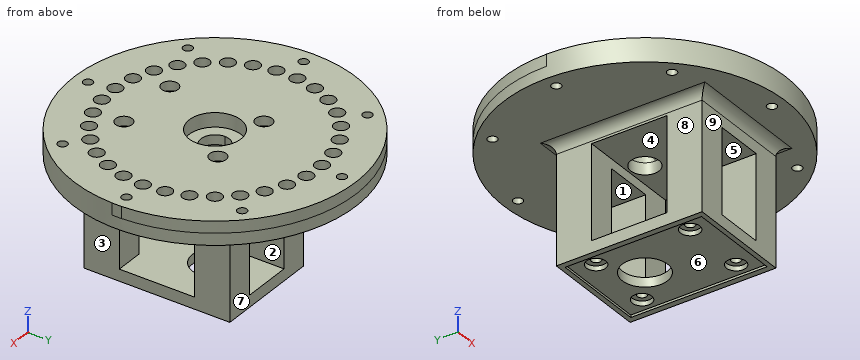
from build123d import *

# Parameters (mm, degrees)
SKETCH1_R               = 3
SKETCH1_R_2             = 11
BOSS_EXTRUDE1_DEPTH     = 5
BOSS_EXTRUDE2_START     = 5
SKETCH2_R               = 60
SKETCH2_R_2             = 6
BOSS_EXTRUDE2_DEPTH     = 5
SKETCH3_R               = 2
CUT_EXTRUDE1_DEPTH      = 35
CUT_EXTRUDE2_START      = -1
SKETCH4_R               = 11
CUT_EXTRUDE2_DEPTH      = 1
CUT_EXTRUDE3_DEPTH      = 87.852680842
CUT_EXTRUDE3_DEPTH_BACK = 87.852680842
SKETCH5_R               = 2
SKETCH6_W               = 45
SKETCH6_H               = 62
BOSS_EXTRUDE3_DEPTH     = 50
CUT_EXTRUDE4_START      = -40
SKETCH7_R               = 2
SKETCH7_R_2             = 6
CUT_EXTRUDE4_DEPTH      = 40
CUT_EXTRUDE5_DEPTH      = 88
CUT_EXTRUDE5_DEPTH_BACK = 5
SKETCH8_R               = 9.6
SKETCH9_W               = 40
SKETCH9_H               = 32
CUT_EXTRUDE6_DEPTH      = 71
SKETCH10_R              = 3.5
CUT_EXTRUDE7_DEPTH      = 4
FILLET1_R               = 4
SKETCH11_W              = 40
SKETCH11_H              = 58
CUT_EXTRUDE8_DEPTH      = 1
SKETCH12_W              = 21
SKETCH12_H              = 36
CUT_EXTRUDE9_DEPTH      = 88
CUT_EXTRUDE10_START     = -88
SKETCH13_R              = 2
CUT_EXTRUDE10_DEPTH     = 88
CUT_EXTRUDE11_START     = -10
SKETCH14_R              = 82.644594736
SKETCH14_R_2            = 60
CUT_EXTRUDE11_DEPTH     = 10
SKETCH15_R              = 4.1
CUT_EXTRUDE12_DEPTH     = 2


with BuildPart() as part:
    # Sketch1 → Boss-Extrude1 (new body)
    with BuildSketch(Plane.XY):
        with BuildLine():
            ThreePointArc((59.966830941, 1.994789941), (-60, 0), (59.966830941, -1.994789941))
            ThreePointArc((59.966830941, -1.994789941), (61.995065687, 0), (59.966830941, 1.994789941))
        make_face()
        with Locations((44, 0)):
            Circle(SKETCH1_R, mode=Mode.SUBTRACT)
        with Locations((43.099317415, -8.857134884)):
            Circle(SKETCH1_R, mode=Mode.SUBTRACT)
        with Locations((40.434143711, -17.351657625)):
            Circle(SKETCH1_R, mode=Mode.SUBTRACT)
        with Locations((36.113591413, -25.135801464)):
            Circle(SKETCH1_R, mode=Mode.SUBTRACT)
        with Locations((30.314544439, -31.890882638)):
            Circle(SKETCH1_R, mode=Mode.SUBTRACT)
        with Locations((23.274416454, -37.34034733)):
            Circle(SKETCH1_R, mode=Mode.SUBTRACT)
        with Locations((15.281431125, -41.261093814)):
            Circle(SKETCH1_R, mode=Mode.SUBTRACT)
        with Locations((6.66282221, -43.49260627)):
            Circle(SKETCH1_R, mode=Mode.SUBTRACT)
        with Locations((-2.228563429, -43.943526316)):
            Circle(SKETCH1_R, mode=Mode.SUBTRACT)
        with Locations((-11.028711419, -42.59539323)):
            Circle(SKETCH1_R, mode=Mode.SUBTRACT)
        with Locations((-19.377342669, -39.503399741)):
            Circle(SKETCH1_R, mode=Mode.SUBTRACT)
        with Locations((-26.932663232, -34.794132425)):
            Circle(SKETCH1_R, mode=Mode.SUBTRACT)
        with Locations((-33.385357398, -28.66038924)):
            Circle(SKETCH1_R, mode=Mode.SUBTRACT)
        with Locations((-38.47125111, -21.353286351)):
            Circle(SKETCH1_R, mode=Mode.SUBTRACT)
        with Locations((-41.982127282, -13.171977411)):
            Circle(SKETCH1_R, mode=Mode.SUBTRACT)
        with Locations((-43.774250229, -4.451406167)):
            Circle(SKETCH1_R, mode=Mode.SUBTRACT)
        with Locations((-43.774250229, 4.451406167)):
            Circle(SKETCH1_R, mode=Mode.SUBTRACT)
        with Locations((-41.982127282, 13.171977411)):
            Circle(SKETCH1_R, mode=Mode.SUBTRACT)
        with Locations((-38.47125111, 21.353286351)):
            Circle(SKETCH1_R, mode=Mode.SUBTRACT)
        with Locations((-33.385357398, 28.66038924)):
            Circle(SKETCH1_R, mode=Mode.SUBTRACT)
        with Locations((-26.932663232, 34.794132425)):
            Circle(SKETCH1_R, mode=Mode.SUBTRACT)
        with Locations((-19.377342669, 39.503399741)):
            Circle(SKETCH1_R, mode=Mode.SUBTRACT)
        with Locations((-11.028711419, 42.59539323)):
            Circle(SKETCH1_R, mode=Mode.SUBTRACT)
        with Locations((-2.228563429, 43.943526316)):
            Circle(SKETCH1_R, mode=Mode.SUBTRACT)
        with Locations((6.66282221, 43.49260627)):
            Circle(SKETCH1_R, mode=Mode.SUBTRACT)
        with Locations((15.281431125, 41.261093814)):
            Circle(SKETCH1_R, mode=Mode.SUBTRACT)
        with Locations((23.274416454, 37.34034733)):
            Circle(SKETCH1_R, mode=Mode.SUBTRACT)
        with Locations((30.314544439, 31.890882638)):
            Circle(SKETCH1_R, mode=Mode.SUBTRACT)
        with Locations((36.113591413, 25.135801464)):
            Circle(SKETCH1_R, mode=Mode.SUBTRACT)
        with Locations((40.434143711, 17.351657625)):
            Circle(SKETCH1_R, mode=Mode.SUBTRACT)
        with Locations((43.099317415, 8.857134884)):
            Circle(SKETCH1_R, mode=Mode.SUBTRACT)
        Circle(SKETCH1_R_2, mode=Mode.SUBTRACT)
    extrude(amount=BOSS_EXTRUDE1_DEPTH)

    # Sketch2 → Boss-Extrude2 (add)
    with BuildSketch(Plane(origin=(0, 0, 0), x_dir=(-1, 0, 0), z_dir=(0, 0, -1)).offset(BOSS_EXTRUDE2_START)):
        Circle(SKETCH2_R)
        Circle(SKETCH2_R_2, mode=Mode.SUBTRACT)
    extrude(amount=-BOSS_EXTRUDE2_DEPTH)

    # Sketch3 → Cut-Extrude1 (cut)
    with BuildSketch(Plane.XY.offset(5)):
        with Locations((0, 54)):
            Circle(SKETCH3_R)
        with Locations((38.183766184, 38.183766184)):
            Circle(SKETCH3_R)
        with Locations((54, 0)):
            Circle(SKETCH3_R)
        with Locations((38.183766184, -38.183766184)):
            Circle(SKETCH3_R)
        with Locations((0, -54)):
            Circle(SKETCH3_R)
        with Locations((-38.183766184, -38.183766184)):
            Circle(SKETCH3_R)
        with Locations((-54, 0)):
            Circle(SKETCH3_R)
        with Locations((-38.183766184, 38.183766184)):
            Circle(SKETCH3_R)
    extrude(amount=-CUT_EXTRUDE1_DEPTH, mode=Mode.SUBTRACT)

    # Sketch4 → Cut-Extrude2 (cut)
    with BuildSketch(Plane.XY.offset(CUT_EXTRUDE2_START)):
        Circle(SKETCH4_R)
    extrude(amount=CUT_EXTRUDE2_DEPTH, mode=Mode.SUBTRACT)

    # Sketch5 → Cut-Extrude3 (cut, two sides: drawn at the far end of the back side and taken through both)
    with BuildSketch(Plane(origin=(0, 0, -5), x_dir=(-1, 0, 0), z_dir=(0, 0, -1)).offset(-CUT_EXTRUDE3_DEPTH_BACK)):
        with Locations((-14, 11)):
            Circle(SKETCH5_R)
        with Locations((14, 11)):
            Circle(SKETCH5_R)
        with Locations((14, -29)):
            Circle(SKETCH5_R)
        with Locations((-14, -29)):
            Circle(SKETCH5_R)
    extrude(amount=CUT_EXTRUDE3_DEPTH + CUT_EXTRUDE3_DEPTH_BACK, mode=Mode.SUBTRACT)

    # Sketch6 → Boss-Extrude3 (add)
    with BuildSketch(Plane(origin=(0, 0, -5), x_dir=(-1, 0, 0), z_dir=(0, 0, -1))):
        with Locations((0, -9)):
            Rectangle(SKETCH6_W, SKETCH6_H)
    extrude(amount=BOSS_EXTRUDE3_DEPTH)

    # Sketch7 → Cut-Extrude4 (cut)
    with BuildSketch(Plane.XY.offset(5).offset(CUT_EXTRUDE4_START)):
        with Locations((-14, 11)):
            Circle(SKETCH7_R)
        with Locations(Location((14, 11, 0), (0, 0, 180))):
            Circle(SKETCH7_R)
        with Locations((14, -29)):
            Circle(SKETCH7_R)
        with Locations(Location((-14, -29, 0), (0, 0, 180))):
            Circle(SKETCH7_R)
        Circle(SKETCH7_R_2)
    extrude(amount=CUT_EXTRUDE4_DEPTH, mode=Mode.SUBTRACT)

    # Sketch8 → Cut-Extrude5 (cut, two sides: drawn at the far end of the back side and taken through both)
    with BuildSketch(Plane(origin=(0, 0, -55), x_dir=(-1, 0, 0), z_dir=(0, 0, -1)).offset(-CUT_EXTRUDE5_DEPTH_BACK)):
        Circle(SKETCH8_R)
    extrude(amount=CUT_EXTRUDE5_DEPTH + CUT_EXTRUDE5_DEPTH_BACK, mode=Mode.SUBTRACT)

    # Sketch9 → Cut-Extrude6 (cut)
    with BuildSketch(Plane.ZY.offset(22.5)):
        with Locations((-30, -9)):
            Rectangle(SKETCH9_W, SKETCH9_H)
    extrude(amount=-CUT_EXTRUDE6_DEPTH, mode=Mode.SUBTRACT)

    # Sketch10 → Cut-Extrude7 (cut)
    with BuildSketch(Plane.XY.offset(5)):
        with Locations((-14, 11)):
            Circle(SKETCH10_R)
        with Locations((14, 11)):
            Circle(SKETCH10_R)
        with Locations((-14, -29)):
            Circle(SKETCH10_R)
        with Locations((14, -29)):
            Circle(SKETCH10_R)
    extrude(amount=-CUT_EXTRUDE7_DEPTH, mode=Mode.SUBTRACT)

    # Fillet1
    fillet1_edges = [part.edges().sort_by_distance(p)[0] for p in [
        (-22.5, -9, -5),
        (0, 22, -5),
        (22.5, -9, -5),
        (0, -40, -5),
    ]]
    fillet(fillet1_edges, radius=FILLET1_R)

    # Sketch11 → Cut-Extrude8 (cut)
    with BuildSketch(Plane(origin=(0, 0, -55), x_dir=(-1, 0, 0), z_dir=(0, 0, -1))):
        with Locations((0, -9)):
            Rectangle(SKETCH11_W, SKETCH11_H)
    extrude(amount=-CUT_EXTRUDE8_DEPTH, mode=Mode.SUBTRACT)

    # Sketch12 → Cut-Extrude9 (cut)
    with BuildSketch(Plane.XZ.offset(40)):
        with Locations((0, -32)):
            Rectangle(SKETCH12_W, SKETCH12_H)
    extrude(amount=-CUT_EXTRUDE9_DEPTH, mode=Mode.SUBTRACT)

    # Sketch13 → Cut-Extrude10 (cut)
    with BuildSketch(Plane.XY.offset(1).offset(CUT_EXTRUDE10_START)):
        with Locations(Location((-14, 11, 0), (0, 0, 180))):
            Circle(SKETCH13_R)
        with Locations(Location((14, 11, 0), (0, 0, 180))):
            Circle(SKETCH13_R)
        with Locations(Location((14, -29, 0), (0, 0, 180))):
            Circle(SKETCH13_R)
        with Locations(Location((-14, -29, 0), (0, 0, 180))):
            Circle(SKETCH13_R)
    extrude(amount=CUT_EXTRUDE10_DEPTH, mode=Mode.SUBTRACT)

    # Sketch14 → Cut-Extrude11 (cut)
    with BuildSketch(Plane.XY.offset(5).offset(CUT_EXTRUDE11_START)):
        Circle(SKETCH14_R)
        with Locations(Location((0, 0, 0), (0, 0, 180))):
            Circle(SKETCH14_R_2, mode=Mode.SUBTRACT)
    extrude(amount=CUT_EXTRUDE11_DEPTH, mode=Mode.SUBTRACT)

    # Sketch15 → Cut-Extrude12 (cut)
    with BuildSketch(Plane(origin=(0, 0, -54), x_dir=(-1, 0, 0), z_dir=(0, 0, -1))):
        with Locations((14, 11)):
            Circle(SKETCH15_R)
        with Locations((-14, 11)):
            Circle(SKETCH15_R)
        with Locations((-14, -29)):
            Circle(SKETCH15_R)
        with Locations((14, -29)):
            Circle(SKETCH15_R)
    extrude(amount=-CUT_EXTRUDE12_DEPTH, mode=Mode.SUBTRACT)


solid = part.part
Work out the finished part from the listing and answer in its coordinate system (mm). Face numbers are marked on the shaded views. A direction names the side the tool comes from. Give positions to 0.01 mm unless a question says otherwise; leave off trailing zeros. Order: outer loops, then holes, each group sorted by start corner. A loop starts at its lowest first (then second) coordinate and runs counter-clockwise, first axis right, second up. Notation, with made-up numbers: (81.25, 15) -> (133.25, 15) arc R26 cw to (133.25, 50) -> close; hole circle Ø4 at (86.5, -14.75). An arc over 180 degrees is marked (long way). One line per item, written item: value.
Item 1: Find section A-A, the plane z = -37. Give the vertices of the cut face in (x, y), plus the area to 3 significant figures.
Answer sheet:
outline: (-22.5, -40) -> (-10.5, -40) -> (-10.5, -25) -> (-22.5, -25) -> close; (-22.5, 7) -> (-10.5, 7) -> (-10.5, 22) -> (-22.5, 22) -> close; (10.5, -40) -> (22.5, -40) -> (22.5, -25) -> (10.5, -25) -> close; (10.5, 7) -> (22.5, 7) -> (22.5, 22) -> (10.5, 22) -> close; hole circle Ø4 at (-14, -29); hole circle Ø4 at (-14, 11); hole circle Ø4 at (14, -29); hole circle Ø4 at (14, 11)
area: 670 mm²
Item 2: Find section D-D, the plane z = -7. Give the vertices of the cut face in (x, y), plus the area to 3 significant figures.
Answer sheet:
outline: (-23.04, -40.54) -> (23.04, -40.54) -> (23.04, 22.54) -> (-23.04, 22.54) -> close; hole circle Ø4 at (-14, -29); hole circle Ø4 at (-14, 11); hole circle Ø12 at (0, 0); hole circle Ø4 at (14, -29); hole circle Ø4 at (14, 11)
area: 2,740 mm²
Item 3: Straight lines are drawn through the part: probe 1 along Y at (x, z) = (-14, -26); probe 2 along Y at (x, z) = (-20.5, -37); probe 3 along Z at (x, y) = (-6, -24). For each, find the intervals that lie inside material, in ascending order.
Answer sheet:
probe 1: -40 to -31, -27 to -25, 7 to 9, 13 to 22
probe 2: -40 to -25, 7 to 22
probe 3: -54 to -50, -10 to 5
Item 4: Find section B-B, the plane x = 54. Give the vertices of the cut face in (y, z), plus the area to 3 significant figures.
Answer sheet:
outline: (-26.15, -5) -> (-2, -5) -> (-2, 5) -> (-26.15, 5) -> close; (2, -5) -> (26.15, -5) -> (26.15, 5) -> (2, 5) -> close
area: 483 mm²
Item 5: Flat-ended cylindrical pins translate along their axes: P1, Ø4.5, axis at x = 54, y = 0, coming from the +Z side; P2, Ø3, axis at x = -26, y = -35, coming from the +Z side; P3, Ø4, axis at y = -38, z = -42, coming from the -X side; P4, Ø20, axis at x = -11, z = -22.5, coming from the -Y side. Find the tip coordinate at first contact, or state that the pin passes through.
Answer sheet:
P1: z = 5
P2: z = 0
P3: x = -22.5
P4: y = -40
Item 6: Determine the mould class of the marked faces 1, 2, 3 and 4 for opening direction X: released by +X, released by -X, zero draft, split by the parting line, or undercut.
Answer sheet:
face 1: undercut
face 2: undercut
face 3: released by +X
face 4: zero draft
Item 7: A tool of negligible diameter and unlimited length cuts with its end or side. For the marked faces 5, 6, 7, 8 and 9, from which of +Z, -Z, +X, -X, +Y, -Y can it reach the whole face along a straight path? Write none if from no direction.
Answer sheet:
face 5: +Y, -Y
face 6: -Z
face 7: -Z, +X, -X, +Y
face 8: -Z, -X, +Y, -Y
face 9: -Z, +X, -X, -Y
